For this review, take the finished solid that the model builds, in its own axes (mm). A direction names the side the tool comes from. Coordinates: 2 decimals unless noted, no trailing zeros. Order: outer loops, then holes, each group sorted by start corner. A loop starts at its lowest first (then second) coordinate and runs counter-clockwise, first axis right, second up. Notation, with made-up numbers: (-22, 58.25) -> (0, 58.25) arc R18 ccw to (0, 82.25) -> close; hole circle Ø8 at (-16, 12). An arc over 180 degrees is marked (long way). Return JSON: item names as keys, results as strings. Group by question number.
Item 1: Take a section at C-C (z = 57). Write out the cut boundary in (x, y) (3 decimals).
Item 2: Draft analysis for pull direction X (two halves, no side actions). For faces 4 (the flat face through (111.125, 0, 52)), 5 (the cylindrical face through (45.81, -0.356, 38.397)), 6 (the flat face through (-1, -1, -9.525)), 7 (the flat face through (60.325, 0, 64)), state which applies: +X half, -X half, draft (parallel to the pull), parting line (faces both ways), or undercut.
Item 3: Take a section at B-B (x = 36.5). Write out the cut boundary in (y, z) (3 decimals), then the cut area to 3 significant figures.
Item 4: Take a section at A-A (y = 3). Write out the cut boundary in (x, z) (3 decimals), then the cut area to 3 significant figures.
Item 5: Machinability: for faces 1 (the flat face through (85, 0, 38.1)), 2 (the flat face through (66, 25.4, 45)), 3 (the flat face through (66, -25.4, 45)), which of the approach directions +Z, -Z, +X, -X, +Y, -Y give a long, thin tool a straight path to every point of the face, cutting with its end or side? Answer none if there is none.
Item 6: Take a section at D-D (x = -18.5). Write out the cut boundary in (y, z) (3 decimals), then the cut area to 3 significant figures.
Item 7: For line 1 along Z through (x, y) = (-6.5, -24) (3 decimals); line 2 along X through (y, z) = (-8, 3) (3 decimals); line 3 along X through (y, z) = (8.5, 63.5) (3 decimals), list the stretches that pass through material, from the lowest coordinate up.
Item 8: Insertion check: pin 1 (2.5 mm diameter, centred on y = 7.5, z = 40, fed in from -X); pin 2 (17 mm diameter, centred on x = 58, z = 39, fed in from +Y); pin 3 (4 mm diameter, centred on y = 19, z = 7.5, fed in from +X) (3 decimals). Each pin has a flat end and moves straight along its axis. Give the tip position at first contact, or say it passes through.
```python
from build123d import *

# Parameters (mm, degrees)
F1_DEPTH = 63.5
F0_W     = 25.4
F0_H     = 19.05
F0_H_2   = 4.7752
F0_H_3   = 4.7498
F2_DEPTH = 25.4


# Not quite as in the source:
# - a feature of the source that left no trace in its solid (it failed there, or was rolled back) is left out


with BuildPart() as f1:
    # F0 (on Front) → F1 (new body, symmetric)
    with BuildSketch(Plane.XZ):
        Polygon((41.275, -9.525), (41.275, 9.525), (22.2228064707, 9.525), (-41.275, 9.525), (-41.275, -9.525), align=None)
    extrude(amount=F1_DEPTH, both=True)

    # F0 (on Front) → F2 (join, symmetric)
    with BuildSketch(Plane.XZ):
        with BuildLine():
            add(Edge.make_bspline(
                [(51.4118423464, 61.5169892273), (53.7469843796, 61.749049716), (56.003883812, 61.8875588148), (58.1631200711, 61.9252)],
                knots=[105.6886926289, 105.6886926289, 105.6886926289, 105.6886926289, 112.3998251036, 112.3998251036, 112.3998251036, 112.3998251036], degree=3))
            ThreePointArc((58.1631200711, 61.9252), (54.7775761271, 61.8849118409), (51.4118423464, 61.5169892273))
        make_face()
        Polygon((41.275, -9.525), (41.275, 9.525), (22.2228064707, 9.525), (-41.275, 9.525), (-41.275, -9.525), align=None)
        with BuildLine():
            Line((41.275, 9.525), (41.0106324272, 26.945333009))
            ThreePointArc((41.0106324272, 26.945333009), (45.9404876374, 38.5224332318), (57.7466785314, 42.8752))
            Line((57.7466785314, 42.8752), (60.325, 42.8752))
            Line((60.325, 42.8752), (60.325, 61.9252))
            Line((60.325, 61.9252), (58.1631200711, 61.9252))
            add(Edge.make_bspline(
                [(51.4118423464, 61.5169892273), (53.7469843796, 61.749049716), (56.003883812, 61.8875588148), (58.1631200711, 61.9252)],
                knots=[105.6886926289, 105.6886926289, 105.6886926289, 105.6886926289, 112.3998251036, 112.3998251036, 112.3998251036, 112.3998251036], degree=3))
            ThreePointArc((51.4118423464, 61.5169892273), (30.2314207387, 49.5916736898), (21.9616330248, 26.7348580473))
            Line((21.9616330248, 26.7348580473), (22.2228064707, 9.525))
            Line((22.2228064707, 9.525), (41.275, 9.525))
        make_face()
        with Locations((73.025, 52.4002)):
            Rectangle(F0_W, F0_H)
        with Locations((73.025, 40.4876)):
            Rectangle(F0_W, F0_H_2)
        Polygon((85.725, 61.9252), (85.725, 42.8752), (85.725, 38.1), (111.125, 38.1), (111.125, 66.675), (85.725, 66.675), align=None)
        with Locations((73.025, 64.3001)):
            Rectangle(F0_W, F0_H_3)
    extrude(amount=F2_DEPTH, both=True)


solid = f1.part
```
Findings below:
{
 "1": {"outline": "(38.964, -25.4) -> (111.125, -25.4) -> (111.125, 25.4) -> (38.964, 25.4) -> close"},
 "2": {"face 4": "+X half", "face 5": "undercut", "face 6": "draft", "face 7": "-X half"},
 "3": {"outline": "(-63.5, -9.525) -> (63.5, -9.525) -> (63.5, 9.525) -> (25.4, 9.525) -> (25.4, 55.382) -> (-25.4, 55.382) -> (-25.4, 9.525) -> (-63.5, 9.525) -> close", "area": "4,750 mm2"},
 "4": {"outline": "(-41.275, -9.525) -> (41.275, -9.525) -> (41.275, 9.525) -> (41.011, 26.945) arc R15.875 cw to (57.747, 42.875) -> (60.325, 42.875) -> (60.325, 38.1) -> (111.125, 38.1) -> (111.125, 66.675) -> (60.325, 66.675) -> (60.325, 61.925) -> (58.163, 61.925) arc R34.925 ccw to (21.962, 26.735) -> (22.223, 9.525) -> (-41.275, 9.525) -> close", "area": "4,180 mm2"},
 "5": {"face 1": "-Z, +X, +Y, -Y", "face 2": "+Z, +X, -X, +Y", "face 3": "+Z, +X, -X, -Y"},
 "6": {"outline": "(-63.5, -9.525) -> (63.5, -9.525) -> (63.5, 9.525) -> (-63.5, 9.525) -> close", "area": "2,420 mm2"},
 "7": {"line 1": "z = -9.525 to 9.525", "line 2": "x = -41.275 to 41.275", "line 3": "x = 60.325 to 111.125"},
 "8": {"pin 1": "stops at x = 23.99", "pin 2": "stops at y = 25.4", "pin 3": "stops at x = 41.275"}
}
